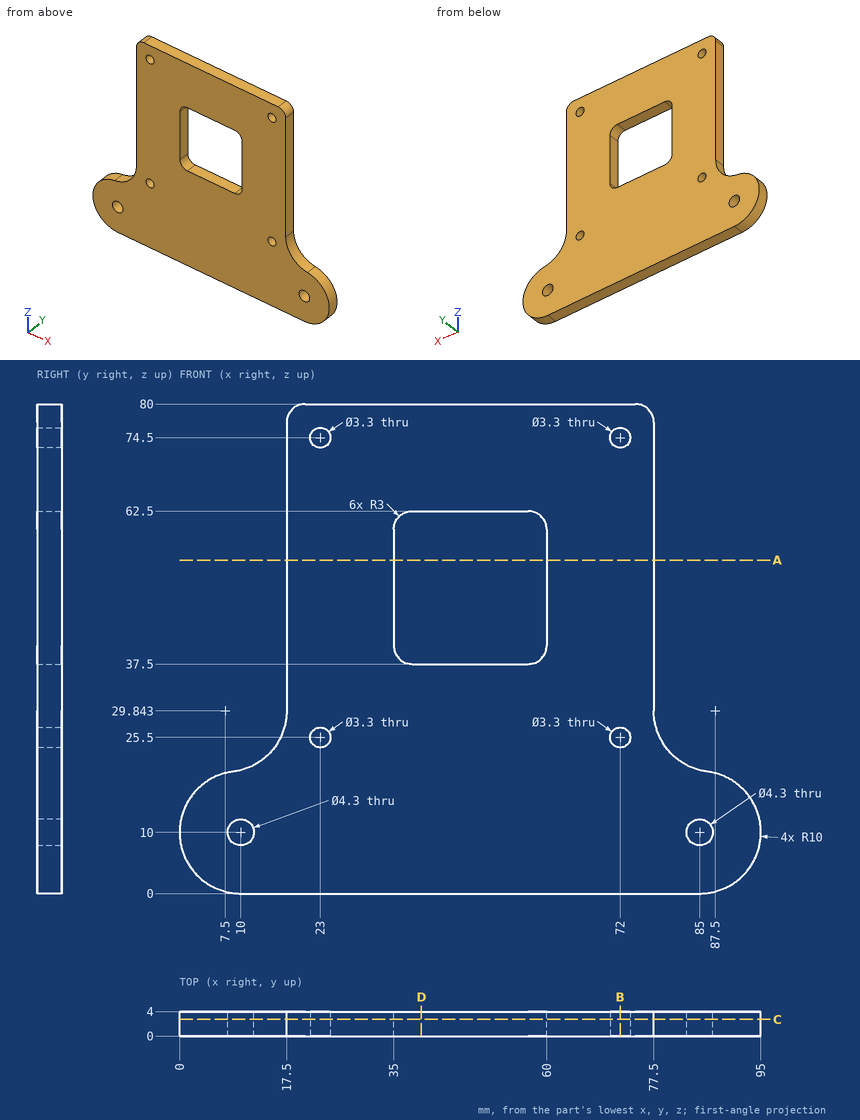
Geometry: see drawing. Coordinates: mm, zero at the bounding-box minimum. Round coordinates to 2 decimals unless told otherwise and drop trailing zeros. Write each loop counter-clockwise with the first axis right and the second up, starting at its lowest first coordinate (ties: lowest second). Pieces come first, ordered by that corner, then holes.
1) Cut plane A-A (z = 54.5). Return the cut outline in (x, y), then the cut area to 3 significant figures.
2) Ray query, L1, parallel to X at y = 1.5, z = 10; L2, parallel to X at y = 1.1, z = 74.5; L3, parallel to Z at x = 39.5, y = 0.85. Return the intervals inside material, ascending.
3) Cut plane B-B (x = 72). Return the cut outline in (y, z), then the cut area to 3 significant figures.
4) Cut plane C-C (y = 2.7). Return the cut outline in (x, z), then the cut area to 3 significant figures.
5) Cut plane D-D (x = 39.5). Return the cut outline in (y, z).
6) Contact query for flat-ended pins moving along their axis: P1, Ø4, axis at x = 72, z = 74.5, coming from the +Y side; P2, Ø1.2, axis at y = 2, z = 64, coming from the +X side; P3, Ø1.2, axis at y = 2.5, z = 49.5, coming from the -X side. Output: stop coordinate, or through.
Geometry says:
1. outline: (17.5, 0) - (35, 0) - (35, 4) - (17.5, 4) - close; (60, 0) - (77.5, 0) - (77.5, 4) - (60, 4) - close
1. area: 140 mm2
2. L1: x = 0 to 7.85, 12.15 to 82.85, 87.15 to 95
2. L2: x = 17.5 to 21.35, 24.65 to 70.35, 73.65 to 77.5
2. L3: z = 0 to 37.5, 62.5 to 80
3. outline: (0, 0) - (4, 0) - (4, 23.85) - (0, 23.85) - close; (0, 27.15) - (4, 27.15) - (4, 72.85) - (0, 72.85) - close; (0, 76.15) - (4, 76.15) - (4, 80) - (0, 80) - close
3. area: 294 mm2
4. outline: (8.75, 19.92) arc R10 ccw to (10, 0) - (85, 0) arc R10 ccw to (86.25, 19.92) arc R10 cw to (77.5, 29.84) - (77.5, 77) arc R3 ccw to (74.5, 80) - (20.5, 80) arc R3 ccw to (17.5, 77) - (17.5, 29.84) arc R10 cw to start; hole circle Ø4.3 at (10, 10); hole circle Ø3.3 at (23, 25.5); hole circle Ø3.3 at (23, 74.5); hole (35, 40.5) arc R3 ccw to (38, 37.5) - (57, 37.5) arc R3 ccw to (60, 40.5) - (60, 59.5) arc R3 ccw to (57, 62.5) - (38, 62.5) arc R3 ccw to (35, 59.5) - close; hole circle Ø3.3 at (72, 25.5); hole circle Ø3.3 at (72, 74.5); hole circle Ø4.3 at (85, 10)
4. area: 4,770 mm2
5. outline: (0, 0) - (4, 0) - (4, 37.5) - (0, 37.5) - close; (0, 62.5) - (4, 62.5) - (4, 80) - (0, 80) - close
6. P1: stops at y = 4
6. P2: stops at x = 77.5
6. P3: stops at x = 17.5
